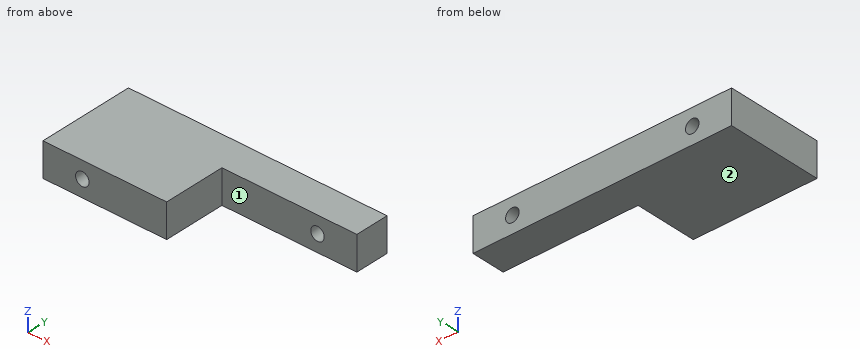
```python
from build123d import *

# Parameters (mm, degrees)
SKETCH1_W                      = 115
SKETCH1_H                      = 15
BOSS_EXTRUDE1_DEPTH            = 42.5
SKETCH2_R                      = 3
CUT_EXTRUDE1_DEPTH             = 42.5
CUT_EXTRUDE2_REACH             = 17
SKETCH3_W                      = 60
SKETCH3_H                      = 27.5
CUT_EXTRUDE2_DIRECTION_2_DEPTH = 1


with BuildPart() as part:
    # Sketch1 → Boss-Extrude1 (new body)
    with BuildSketch(Plane(origin=(0, 0, 0), x_dir=(1, 0, 0), z_dir=(0, 1, 0))):
        Rectangle(SKETCH1_W, SKETCH1_H)
    extrude(amount=BOSS_EXTRUDE1_DEPTH)

    # Sketch2 → Cut-Extrude1 (cut)
    with BuildSketch(Plane(origin=(0, 42.5, 0), x_dir=(1, 0, 0), z_dir=(0, 1, 0))):
        with Locations((-40, 0)):
            Circle(SKETCH2_R)
        with Locations((40, 0)):
            Circle(SKETCH2_R)
    extrude(amount=-CUT_EXTRUDE1_DEPTH, mode=Mode.SUBTRACT)

    # Sketch3 → Cut-Extrude2 (cut, up to next)
    with BuildSketch(Plane.XY.offset(7.5), mode=Mode.PRIVATE) as cut_extrude2_sk1:
        with Locations((27.5, 13.75)):
            Rectangle(SKETCH3_W, SKETCH3_H)
    cut_extrude2_tool1 = extrude(cut_extrude2_sk1.sketch, amount=-CUT_EXTRUDE2_REACH, mode=Mode.PRIVATE) & part.part
    add(cut_extrude2_tool1.solids().sort_by_distance((27.5, 13.75, 7.5))[0], mode=Mode.SUBTRACT)

    # Sketch3 → Cut-Extrude2 direction 2 (cut)
    with BuildSketch(Plane.XY.offset(7.5)):
        with Locations((27.5, 13.75)):
            Rectangle(SKETCH3_W, SKETCH3_H)
    extrude(amount=CUT_EXTRUDE2_DIRECTION_2_DEPTH, mode=Mode.SUBTRACT)


solid = part.part
```
Verification items for the finished model (mm, model axes). Face numbers are marked on the shaded views. A direction names the side the tool comes from. Give positions to 0.01 mm unless a question says otherwise; leave off trailing zeros. Loops run counter-clockwise (first coordinate to the right, second up) from the corner with the lowest first, then second, coordinate; pieces in that order, holes last.
1. Section check B-B, the plane z = 0. Enter the section's corners in (x, y).
2. Set-up check for the marked faces 1 and 2: record each of +Z, -Z, +X, -X, +Y, -Y from which the full face is reachable in a straight line by a thin tool's end or side.
3. Section check C-C, the plane y = 24. Enter the section's corners in (x, z).
4. Thickness scan on line 1 (X direction, y = 33, z = 0); line 2 (X direction, y = 13, z = 0); line 3 (Z direction, x = 40, y = 39.75). Record the ranges inside material, lowest first.
5. Section check D-D, the plane x = 40. Enter the section's corners in (y, z).
6. Go/stop test with flat-tipped pins: pin 1 Ø4.5 at (y, z) = (9.5, 0.5) entering from +X; pin 2 Ø8 at (x, z) = (40, 0) entering from -Y. Record where each tip stops, or that it passes through.
7. Section check A-A, the plane x = -40. Enter the section's corners in (y, z), then the cut area to 4 significant figures.
Geometry says:
1. outline: (-57.5, 0) - (-43, 0) - (-43, 42.5) - (-57.5, 42.5) - close; (-37, 0) - (-2.5, 0) - (-2.5, 27.5) - (37, 27.5) - (37, 42.5) - (-37, 42.5) - close; (43, 27.5) - (57.5, 27.5) - (57.5, 42.5) - (43, 42.5) - close
2. face 1: +Z, -Z, +X, -Y
2. face 2: -Z, +X, -X, +Y, -Y
3. outline: (-57.5, -7.5) - (-2.5, -7.5) - (-2.5, 7.5) - (-57.5, 7.5) - close; hole circle Ø6 at (-40, 0)
4. line 1: x = -57.5 to -43, -37 to 37, 43 to 57.5
4. line 2: x = -57.5 to -43, -37 to -2.5
4. line 3: z = -7.5 to -3, 3 to 7.5
5. outline: (27.5, -7.5) - (42.5, -7.5) - (42.5, -3) - (27.5, -3) - close; (27.5, 3) - (42.5, 3) - (42.5, 7.5) - (27.5, 7.5) - close
6. pin 1: stops at x = -2.5
6. pin 2: stops at y = 27.5
7. outline: (0, -7.5) - (42.5, -7.5) - (42.5, -3) - (0, -3) - close; (0, 3) - (42.5, 3) - (42.5, 7.5) - (0, 7.5) - close
7. area: 382.5 mm2
